Autodesk Inventor part; units mm, degrees
ref_plane "YZ Plane" through (0, 0, 0) normal (1, 0, 0) x (0, 1, 0)
ref_plane "XZ Plane" through (0, 0, 0) normal (0, 1, 0) x (-1, 0, 0)
ref_plane "XY Plane" through (0, 0, 0) normal (0, 0, 1) x (1, 0, 0)
sketch "Sketch1" plane through (0, 0, 0) normal (1, 0, 0) x (0, 1, 0)
  circle A0 centre (0, 0) radius 12.7
  arc A1 (12.1376, -3.7374) -> (12.1376, 3.7374) centre (0, 0) ccw
  dimension "d0" = 25.4
extrude "Extrusion1" add sketch "Sketch1" along normal blind 12.7
sketch "Sketch2" plane through (12.7, 0, 0) normal (1, 0, 0) x (0, 0, -1)
  circle A0 centre (0, 0) radius 12.7 construction
  line L0 (0, 12.7) -> (3.175, 12.7) construction
  line L1 (0, 12.7) -> (-3.175, 12.7) construction
  line L2 (-3.175, 12.7) -> (0, 15.875) construction
  line L3 (0, 15.875) -> (3.175, 12.7) construction
  line L4 (0, 15.875) -> (-3.7374, 12.1376)
  line L5 (0, 15.875) -> (3.7374, 12.1376)
  arc A1 (3.7374, 12.1376) -> (-3.7374, 12.1376) centre (0, 0) ccw
  line L6 (-9.3311, 12.8431) -> (-10.1579, 7.6228)
  line L7 (-9.3311, 12.8431) -> (-4.1107, 12.0163)
  arc A2 (-4.1107, 12.0163) -> (-10.1579, 7.6228) centre (0, 0) ccw
  line L8 (-15.098, 4.9056) -> (-12.6985, 0.1963)
  line L9 (-15.098, 4.9056) -> (-10.3887, 7.3052)
  arc A3 (-10.3887, 7.3052) -> (-12.6985, 0.1963) centre (0, 0) ccw
  line L10 (-15.098, -4.9056) -> (-10.3887, -7.3052)
  line L11 (-15.098, -4.9056) -> (-12.6985, -0.1963)
  arc A4 (-12.6985, -0.1963) -> (-10.3887, -7.3052) centre (0, 0) ccw
  line L12 (-9.3311, -12.8431) -> (-4.1107, -12.0163)
  line L13 (-9.3311, -12.8431) -> (-10.1579, -7.6228)
  arc A5 (-10.1579, -7.6228) -> (-4.1107, -12.0163) centre (0, 0) ccw
  line L14 (0, -15.875) -> (3.7374, -12.1376)
  line L15 (0, -15.875) -> (-3.7374, -12.1376)
  arc A6 (-3.7374, -12.1376) -> (3.7374, -12.1376) centre (0, 0) ccw
  line L16 (9.3311, -12.8431) -> (10.1579, -7.6228)
  line L17 (9.3311, -12.8431) -> (4.1107, -12.0163)
  arc A7 (4.1107, -12.0163) -> (10.1579, -7.6228) centre (0, 0) ccw
  line L18 (15.098, -4.9056) -> (12.6985, -0.1963)
  line L19 (15.098, -4.9056) -> (10.3887, -7.3052)
  arc A8 (10.3887, -7.3052) -> (12.6985, -0.1963) centre (0, 0) ccw
  line L20 (15.098, 4.9056) -> (10.3887, 7.3052)
  line L21 (15.098, 4.9056) -> (12.6985, 0.1963)
  arc A9 (12.6985, 0.1963) -> (10.3887, 7.3052) centre (0, 0) ccw
  line L22 (9.3311, 12.8431) -> (4.1107, 12.0163)
  line L23 (9.3311, 12.8431) -> (10.1579, 7.6228)
  arc A10 (10.1579, 7.6228) -> (4.1107, 12.0163) centre (0, 0) ccw
  point P0 (-7.4649, 10.2745)
  point P1 (-12.0784, 3.9245)
  point P2 (-12.0784, -3.9245)
  point P3 (-7.4649, -10.2745)
  point P4 (0, -12.7)
  point P5 (7.4649, -10.2745)
  point P6 (12.0784, -3.9245)
  point P7 (12.0784, 3.9245)
  point P8 (7.4649, 10.2745)
  dimension "d6" = 3.175
  dimension "d7" = 3.175
  dimension "d8" = 45
  dimension "d11" = 360
extrude "Extrusion2" add sketch "Sketch2" against normal blind 12.7
sketch "Sketch3" plane through (12.7, 0, 0) normal (1, 0, 0) x (0, 0, -1)
  circle A0 centre (0, 0) radius 1.905
  dimension "d15" = 3.81
extrude "Extrusion3" cut sketch "Sketch3" against normal blind 6.35
properties part number "Finger Pinion"
Part model, mm, in its own coordinate system. A direction names the side the tool comes from. Give positions to 0.01 mm unless a question says otherwise; leave off trailing zeros. Order: outer loops, then holes, each group sorted by start corner. A loop starts at its lowest first (then second) coordinate and runs counter-clockwise, first axis right, second up. Notation, with made-up numbers: (18, -14) - (60, -14) arc R23 ccw to (60, 9) - close; hole circle Ø3 at (19, 9). An arc over 180 degrees is marked (long way). Use one line per item in the form item = value.
Item 1: Which spindle directions (+Z, -Z, +X, -X, +Y, -Y) get a long thin tool onto all of the face, cutting with end or side? Do faces 4 (the face through (6.439, 2.584, 13.915)), 5 (the face through (6.439, -12.435, 6.757)), 6 (the face through (6.439, -2.584, -13.915)). Say none if no direction does.
Solution:
face_4 = +Z, +X, -X
face_5 = +X, -X, -Y
face_6 = -Z, +X, -X
Item 2: Two-plate mould, pull along Z, no slides. Class faces 1 (the face through (6.439, 2.584, -13.915)), 2 (the face through (9.57, -1.86, 0.41)), 3 (the face through (6.439, 6.089, 12.776)): released by +Z, released by -Z, zero draft, split by the parting line, or undercut.
Solution:
face_1 = released by -Z
face_2 = undercut
face_3 = released by +Z
Item 3: Probe probe 1 along Y at (x, z) = (10, 1.5) (3 decimals); probe 2 along Z at (x, y) = (3, -2); probe 3 along Z at (x, y) = (3.5, 8.5). List the from-to ranges inside material, lowest first. Write a range as from..to.
Solution:
probe_1 = -14.375..-1.174, 1.174..14.375
probe_2 = -13.62..13.62
probe_3 = -10.02..10.02
Item 4: Slice it at B-B on z = -1.5. Give the cut face in (x, y) (3 decimals), and give its area (3 significant figures).
Solution:
outline = (0, -14.375) - (12.7, -14.375) - (12.7, -1.174) - (6.35, -1.174) - (6.35, 1.174) - (12.7, 1.174) - (12.7, 14.375) - (0, 14.375) - close
area = 350 mm2
Item 5: Slice it at D-D on y = -4. Give the cut face in (x, z).
Solution:
outline = (0, -14.64) - (12.7, -14.64) - (12.7, 14.64) - (0, 14.64) - close
Item 6: Pin check, flat tips, straight feed: pin 1 Ø3.5 at (y, z) = (0, 0) entering from +X; pin 2 Ø3 at (x, z) = (8, 5.5) entering from +Y; pin 3 Ø4 at (x, z) = (10, -6.5) entering from +Y. Stop position of each tip, or through.
Solution:
pin_1 = 6.35
pin_2 = 12.47
pin_3 = 12.71
